The drawing under review shows one solid part. Ordinate dimensions are in mm from its lowest x, y, z. A direction names the side the tool comes from. Give positions to 0.01 mm unless a question says otherwise; leave off trailing zeros. Write each loop counter-clockwise with the first axis right and the second up, starting at its lowest first coordinate (ties: lowest second). Pieces come first, ordered by that corner, then holes. Notation, with made-up numbers: M 9,-6 L 58,-6 A10 cw 58,12 Z; hole C 64.25,84.25 d8. An arc over 180 degrees is marked long. Use one line per item in the form item = value. Start each with the question number.
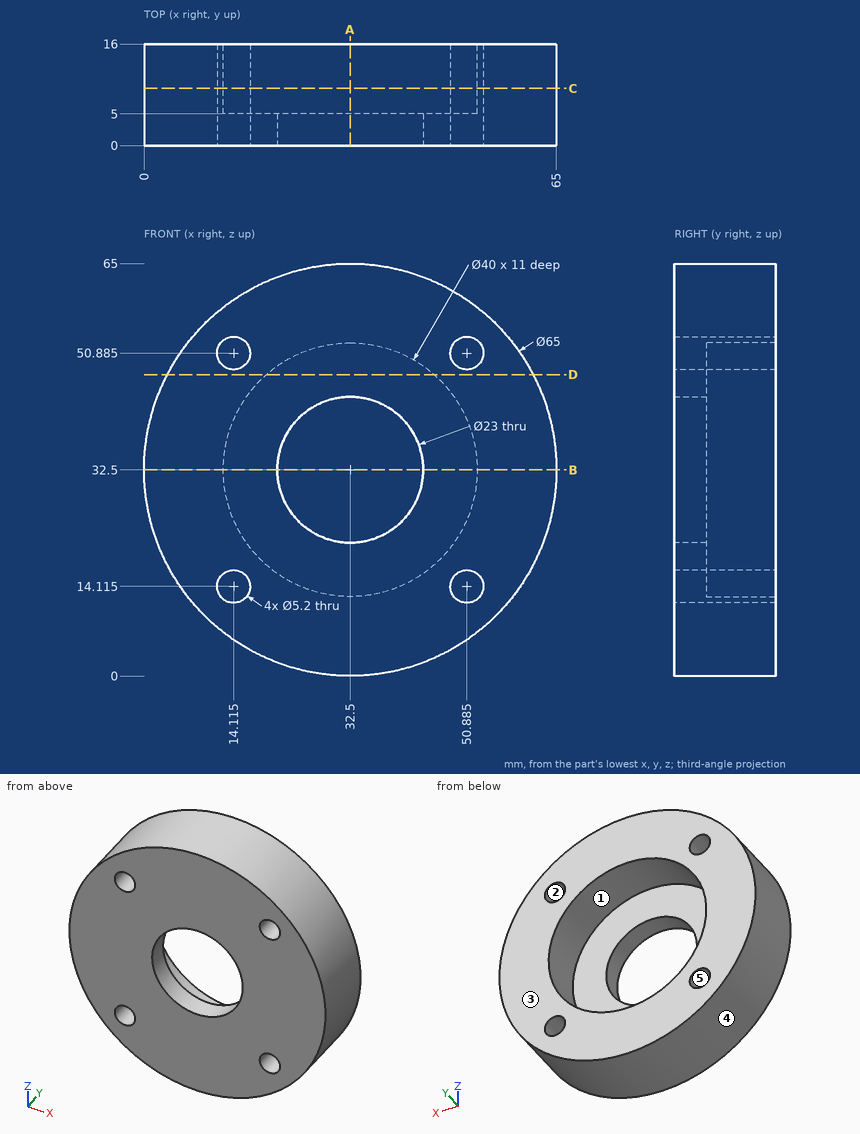
1. For the marked faces 1 and 2, list the 3-axis set-ups (+Z, -Z, +X, -X, +Y, -Y) from which the entire face can be reached by the end or side of a thin tool; tool diameter is ignored.
2. Draft analysis for pull direction Z (two halves, no side actions). For the marked faces 3, 4 and 5, state which applies: pulls with the +Z half, pulls with the -Z half, needs draft (parallel to the pull), parting line crosses it, or undercut.
3. To check wall thickness, follow L1, parallel to Z at x = 49.5, y = 3.5 (1 decimal); L2, parallel to Y at x = 36, z = 46.5; L3, parallel to Z at x = 17, y = 7 (1 decimal). State the ranges of each line that lie inside material, in increasing order.
4. We need section B-B (z = 32.5). State the section outline as (x, y) points.
5. We need section A-A (x = 32.5). State the section outline as (y, z) points, and give its area (3 significant figures).
6. Clearance check with flat-ended pins moving along their axes: pin 1 Ø3 at (y, z) = (4.5, 45) entering from -X; pin 2 Ø6 at (y, z) = (11.5, 7) entering from +X; pin 3 Ø6 at (x, y) = (27, 7) entering from -Z. State where each tip first meets the part, or that it passes through.
7. We need section D-D (z = 47.5). State the section outline as (x, y) points.
8. We need section C-C (y = 9). State the section outline as (x, z) points (1 decimal), and give its area (3 significant figures).
Answer block:
q1.face_1 = +Y
q1.face_2 = +Y, -Y
q2.face_3 = needs draft
q2.face_4 = parting line crosses it
q2.face_5 = undercut
q3.L1 = 4.8 to 11.9, 16.3 to 48.7, 53.1 to 60.2
q3.L2 = 0 to 5
q3.L3 = 3.9 to 19.9, 45.1 to 61.1
q4.outline = M 0,0 L 21,0 L 21,5 L 12.5,5 L 12.5,16 L 0,16 Z; M 44,0 L 65,0 L 65,16 L 52.5,16 L 52.5,5 L 44,5 Z
q5.outline = M 0,0 L 16,0 L 16,12.5 L 5,12.5 L 5,21 L 0,21 Z; M 0,44 L 5,44 L 5,52.5 L 16,52.5 L 16,65 L 0,65 Z
q5.area = 485 mm^2
q6.pin_1 = 1.92
q6.pin_2 = 55.95
q6.pin_3 = 0.1
q7.outline = M 3.67,0 L 61.33,0 L 61.33,16 L 45.73,16 L 45.73,5 L 19.27,5 L 19.27,16 L 3.67,16 Z
q8.outline = C 32.5,32.5 d65; hole C 14.1,14.1 d5.2; hole C 14.1,50.9 d5.2; hole C 32.5,32.5 d40; hole C 50.9,14.1 d5.2; hole C 50.9,50.9 d5.2
q8.area = 1,980 mm^2
